Autodesk Inventor part; units mm, degrees
ref_plane "YZ Plane" through (0, 0, 0) normal (1, 0, 0) x (0, 1, 0)
ref_plane "XZ Plane" through (0, 0, 0) normal (0, 1, 0) x (-1, 0, 0)
ref_plane "XY Plane" through (0, 0, 0) normal (0, 0, 1) x (1, 0, 0)
sketch "スケッチ1" plane through (0, 0, 0) normal (0, 0, 1) x (1, 0, 0)
  line L0 (7.5, -6) -> (-7.5, -6)
  line L1 (-7.5, -6) -> (-7.5, 6)
  line L2 (-7.5, 6) -> (7.5, 6)
  line L3 (7.5, 6) -> (7.5, -6)
  line L4 (7.5, -6) -> (-7.5, 6) construction
  line L5 (-7.5, -6) -> (7.5, 6) construction
  point P0 (0, 0)
  point P1 (0, 0)
  point P2 (0, 0)
  dimension "d2" = 15
  dimension "d4" = 12
extrude "押し出し1" add sketch "スケッチ1" along normal mid plane 33.6
sketch "スケッチ3" plane through (7.5, -6, -16.8) normal (1, 0, 0) x (0, 0, -1)
  line L0 (-29.3, 8.5) -> (-4.3, 8.5)
  line L1 (-4.3, 8.5) -> (-4.3, 3.5)
  line L2 (-4.3, 3.5) -> (-29.3, 3.5)
  line L3 (-29.3, 3.5) -> (-29.3, 8.5)
  line L4 (-29.3, 8.5) -> (-4.3, 3.5) construction
  line L5 (-4.3, 8.5) -> (-29.3, 3.5) construction
  line L6 (-31.3, 12) -> (-29.3, 12)
  line L7 (-29.3, 12) -> (-29.3, 0)
  line L8 (-29.3, 0) -> (-31.3, 0)
  line L9 (-31.3, 0) -> (-31.3, 12)
  line L10 (0, 0) -> (-33.6, 0)
  line L11 (-2.3, 12) -> (-2.3, 0)
  line L12 (-4.3, 0) -> (-4.3, 12)
  line L13 (-2.3, 0) -> (-4.3, 0)
  line L14 (-4.3, 12) -> (-2.3, 12)
  point P0 (-16.8, 6)
  point P1 (-16.8, 6)
  point P2 (-16.8, 6)
  point P3 (-29.3, 6)
  point P4 (-30.3, 0)
  point P5 (-18.35, 0)
  point P6 (-4.3, 6)
  point P7 (-3.3, 12)
  point P8 (-4.3, 3.5)
  dimension "d11" = 25
  dimension "d14" = 12
  dimension "d15" = 2
  dimension "d18" = 360
  dimension "d26" = 5
extrude "押し出し3" cut sketch "スケッチ3" against normal blind 9 contours L0 L1 L2 L3 | L3 L7 L8 L9 L6 | L12 L14 L11 L10 L1
sketch "スケッチ4" plane through (0, 0, -16.8) normal (0, 0, -1) x (-1, 0, 0)
  circle A0 centre (-1.5, 0) radius 3
  line L0 (-7.5, 6) -> (-7.5, -6)
  point P0 (0, 0)
  dimension "d22" = 6
  dimension "d23" = 6
extrude "押し出し4" cut sketch "スケッチ4" against normal up to surface (2.3 mm away)
mirror "ミラー1" about plane through (0, 0, 0) normal (0, 0, 1) of "押し出し4"
sketch "スケッチ5" plane through (-7.5, 6, -16.8) normal (0, 1, 0) x (1, 0, 0)
  line L0 (15, -4.3) -> (15, -29.3)
  line L1 (6, -4.3) -> (15, -4.3)
  line L2 (15, -29.3) -> (11, -29.3)
  line L3 (11, -29.3) -> (11, -4.3)
  line L4 (11, -4.3) -> (15, -4.3)
  line L5 (15, -4.3) -> (15, -29.3)
  line L6 (11, -18.7) -> (3, -18.7)
  line L7 (3, -18.7) -> (3, -14.9)
  line L8 (3, -14.9) -> (11, -14.9)
  line L9 (11, -14.9) -> (11, -18.7)
  point P0 (11, -16.8)
  point P1 (11, -16.8)
  dimension "d30" = 4
  dimension "d36" = 8
  dimension "d37" = 3.8
extrude "押し出し5" cut sketch "スケッチ5" against normal through all
fillet "フィレット4" radius 2 8 edges at (0, 6, -16.8) (0, -6, -16.8) (0, 6, 16.8) (0, -6, 16.8) (3.5, 6, 7.2) (3.5, 6, -7.2) (3.5, -6, -7.2) (3.5, -6, 7.2)
properties part number "Cable_fixing" material "熱可塑性 樹脂"
Read the model definition and answer for the solid it produces. Units are mm, in the model's axes. A direction names the side the tool comes from. Coordinates: 2 decimals unless noted, no trailing zeros. Write each loop counter-clockwise with the first axis right and the second up, starting at its lowest first coordinate (ties: lowest second). Pieces come first, ordered by that corner, then holes. Notation, with made-up numbers: (-5.5, 29) - (52.5, 29) arc R30 ccw to (52.5, 52) - close; hole circle Ø7 at (-25, 41). An arc over 180 degrees is marked (long way). Answer as a JSON object with one key per item and string values. Group by question number.
1. A cutting plane is placed at B-B (z = 3). Determine the outline of the cut face in (x, y), plus the area to 3 significant figures.
2. Which of the six approach directions +Z, -Z, +X, -X, +Y, -Y give full straight-line access (tool end or side, diameter ignored) to faces 4 (the cylindrical face through (2.9, 5.43, -7.27)), 5 (the flat face through (1, -2.5, 7)), 6 (the cylindrical face through (2.9, -5.43, -7.13)), 7 (the flat face through (-5, 6, 0)), 8 (the flat face through (3.5, 3, -7))?
3. A cutting plane is placed at D-D (z = -14). Determine the outline of the cut face in (x, y), plus the area to 3 significant figures.
4. Consider L1, parallel to Z at x = 3.25, y = -3; L2, parallel to Z at x = -2.5, y = 0.25; L3, parallel to Z at x = 4.25, y = -2. Determine where each line is inside the solid, lowest interval first. Write a range as [from, to].
5. The mould has two halves that part along X. Classify faces 1 (the cylindrical face through (2.9, -5.43, 7.27)), 2 (the cylindrical face through (3.9, -1.8, -15.7)), 3 (the flat face through (5, 0, -14.5)): +X half, -X half, draft (parallel to the pull), parting line (faces both ways), or undercut.
6. A cutting plane is placed at C-C (y = 1.5). Determine the outline of the cut face in (x, z).
7. Each of these flat-tipped pins is pushed along its axis until it touches: P1, Ø1.6, axis at y = 3.5, z = 9.5, coming from the +X side; P2, Ø3, axis at y = -0.5, z = -8.5, coming from the +X side; P3, Ø1.9, axis at y = 0, z = 0, coming from the +X side. Where does it stop, or does it pass through?
8. A cutting plane is placed at A-A (x = 5.5). Determine the outline of the cut face in (y, z).
Worked out:
{
 "1": {"outline": "(-7.5, -6) - (1.5, -6) arc R2 ccw to (3.5, -4) - (3.5, -2.5) - (-1.5, -2.5) - (-1.5, 2.5) - (3.5, 2.5) - (3.5, 4) arc R2 ccw to (1.5, 6) - (-7.5, 6) - close", "area": "105 mm²"},
 "2": {"face 4": "+X, +Y", "face 5": "+X", "face 6": "+X, -Y", "face 7": "+Z, -Z, +X, -X, +Y", "face 8": "+X, +Y, -Y"},
 "3": {"outline": "(-7.5, -6) - (-1.5, -6) - (-1.5, 6) - (-7.5, 6) - close", "area": "72.0 mm²"},
 "4": {"L1": "z = [-16.8, -14.5], [-12.5, -1.9], [1.9, 12.5], [14.5, 16.8]", "L2": "z = [-16.8, -1.9], [1.9, 16.8]", "L3": "z = [-16.8, -14.5], [14.5, 16.8]"},
 "5": {"face 1": "+X half", "face 2": "undercut", "face 3": "draft"},
 "6": {"outline": "(-7.5, -16.8) - (-1.1, -16.8) - (-1.1, -14.5) - (-1.5, -14.5) - (-1.5, -1.9) - (-4.5, -1.9) - (-4.5, 1.9) - (-1.5, 1.9) - (-1.5, 14.5) - (-1.1, 14.5) - (-1.1, 16.8) - (-7.5, 16.8) - close; (4.1, -16.8) - (7.5, -16.8) - (7.5, -14.5) - (4.1, -14.5) - close; (4.1, 14.5) - (7.5, 14.5) - (7.5, 16.8) - (4.1, 16.8) - close"},
 "7": {"P1": "stops at x = 3.5", "P2": "stops at x = -1.5", "P3": "stops at x = -4.5"},
 "8": {"outline": "(-6, -14.8) arc R2 ccw to (-4, -16.8) - (4, -16.8) arc R2 ccw to (6, -14.8) - (6, -14.5) - (-6, -14.5) - close; (-6, 14.5) - (6, 14.5) - (6, 14.8) arc R2 ccw to (4, 16.8) - (-4, 16.8) arc R2 ccw to (-6, 14.8) - close"}
}
